Geometry: final body of the model. Coordinates: model frame, mm. A direction names the side the tool comes from. Round coordinates to 2 decimals unless told otherwise and drop trailing zeros. Loops run counter-clockwise (first coordinate to the right, second up) from the corner with the lowest first, then second, coordinate; pieces in that order, holes last. Notation, with made-up numbers: M 74.5,5.25 L 89.5,5.25 A26 ccw 89.5,40.25 Z; hole C 54,12.25 d9. An arc over 180 degrees is marked long. Return JSON: item names as keys, results as strings.
from build123d import *

# Parameters (mm, degrees)
BOSS_EXTRUDE1_DEPTH = 10
BOSS_EXTRUDE2_DEPTH = 10
SKETCH3_R           = 10
BOSS_EXTRUDE3_DEPTH = 382


with BuildPart() as part:
    # Sketch1 → Boss-Extrude1 (new body)
    with BuildSketch(Plane.XY):
        with BuildLine():
            Line((-325, 0), (-70, 0))
            ThreePointArc((-70, 0), (0, 44.921970135), (70, 0))
            Line((70, 0), (325, 0))
            ThreePointArc((325, 0), (269.81612239, 123.213044268), (155, 194.233975444))
            ThreePointArc((155, 194.233975444), (0, 154.921970135), (-155, 194.233975444))
            ThreePointArc((-155, 194.233975444), (-269.81612239, 123.213044268), (-325, 0))
        make_face()
    extrude(amount=BOSS_EXTRUDE1_DEPTH)



with BuildPart() as body_2:
    # Sketch2 → Boss-Extrude2 (new body)
    with BuildSketch(Plane.XY.offset(-362)):
        with BuildLine():
            Line((70, 0), (325, 0))
            ThreePointArc((325, 0), (269.81612239, 123.213044268), (155, 194.233975444))
            ThreePointArc((155, 194.233975444), (0, 154.921970135), (-155, 194.233975444))
            ThreePointArc((-155, 194.233975444), (-269.81612239, 123.213044268), (-325, 0))
            Line((-325, 0), (-70, 0))
            ThreePointArc((-70, 0), (0, 44.921970135), (70, 0))
        make_face()
    extrude(amount=-BOSS_EXTRUDE2_DEPTH)


with BuildPart() as part_1:
    add(part.part)

    add(body_2.part)  # Boss-Extrude3 merges body 2
    # Sketch3 → Boss-Extrude3 (add)
    with BuildSketch(Plane.XY.offset(10)):
        with Locations((-160, 83.10096245)):
            Circle(SKETCH3_R)
        with Locations((160, 83.10096245)):
            Circle(SKETCH3_R)
    extrude(amount=-BOSS_EXTRUDE3_DEPTH)


solid = part_1.part
Q1. Pull-direction query (Z, two-part tool) for faces 1 (the cylindrical face through (271.074, 121.764, 4.93)), 2 (the cylindrical face through (169.237, 79.271, -178.466)), 3 (the flat face through (-5, 77, -372)), 4 (the flat face through (-5, 77, -362)); classes: pulls with the +Z half, pulls with the -Z half, needs draft (parallel to the pull), parting line crosses it, or undercut.
Determined:
{"face 1": "needs draft", "face 2": "undercut", "face 3": "pulls with the -Z half", "face 4": "undercut"}
Q2. Reachability of faces 5 (the cylindrical face through (-150.763, 79.271, -178.466)), 6 (the cylindrical face through (-268.55, 124.65, -366.93)) from +Z, -Z, +X, -X, +Y, -Y: full face, straight path, thin tool, end or side. Return the list, or none.
Determined:
{"face 5": "none", "face 6": "+Z, -Z, -X, +Y"}
Q3. Section query C-C (y = 164). Output: boundary loops of the cut face in (x, z), plus the area to 3 significant figures.
Determined:
{"outline": "M -222.97,-372 L -76.3,-372 L -76.3,-362 L -222.97,-362 Z; M -222.97,0 L -76.3,0 L -76.3,10 L -222.97,10 Z; M 76.3,-372 L 222.97,-372 L 222.97,-362 L 76.3,-362 Z; M 76.3,0 L 222.97,0 L 222.97,10 L 76.3,10 Z", "area": "5,870 mm^2"}
Q4. Section query A-A (x = -276). Output: boundary loops of the cut face in (y, z), plus the area to 3 significant figures.
Determined:
{"outline": "M 0,-372 L 115.84,-372 L 115.84,-362 L 0,-362 Z; M 0,0 L 115.84,0 L 115.84,10 L 0,10 Z", "area": "2,320 mm^2"}
Q5. Section query B-B (y = 64). Output: boundary loops of the cut face in (x, z), plus the area to 3 significant figures.
Determined:
{"outline": "M -307.43,-372 L 307.43,-372 L 307.43,-362 L -307.43,-362 Z; M -307.43,0 L 307.43,0 L 307.43,10 L -307.43,10 Z", "area": "12,300 mm^2"}
Q6. Pin query (flat end, axial travel): pin 1 (3 mm diameter, centred on y = 75.5, z = -222, fed in from -X). Return the tip coordinate at first contact, or that it passes through.
Determined:
{"pin 1": "stops at x = -167.92"}
Q7. Material intervals for L1, parallel to Z at x = 216, y = 84.5; L2, parallel to X at y = 92, z = -225; L3, parallel to X at y = 80, z = -97, sorted ascending.
Determined:
{"L1": "z = -372 to -362, 0 to 10", "L2": "x = -164.56 to -155.44, 155.44 to 164.56", "L3": "x = -169.51 to -150.49, 150.49 to 169.51"}
Q8. Section query D-D (z = -292). Output: boundary loops of the cut face in (x, y).
Determined:
{"outline": "C -160,83.1 d20; C 160,83.1 d20"}
